```python
from build123d import *
from build123d.topology import SkipClean

# Parameters (mm, degrees)
SKETCH1_R           = 40
BOSS_EXTRUDE1_DEPTH = 4
BOSS_EXTRUDE2_DEPTH = 3
CUT_EXTRUDE1_DEPTH  = 3


with BuildPart() as part:
    # Sketch1 → Boss-Extrude1 (new body)
    with BuildSketch(Plane(origin=(0, 0, 0), x_dir=(1, 0, 0), z_dir=(0, 1, 0))):
        with Locations(Location((0, 0, 0), (0, 0, 270))):
            Circle(SKETCH1_R)
    extrude(amount=BOSS_EXTRUDE1_DEPTH)

    # Sketch2 → Boss-Extrude2 (add)
    with SkipClean():  # the faces are left unmerged after this step: merging them gives an invalid solid
        with BuildSketch(Plane(origin=(0, 4, 0), x_dir=(1, 0, 0), z_dir=(0, 1, 0))):
            with BuildLine():
                Line((70.838532525, 75.016207091), (33.556064162, 21.771324213))
                ThreePointArc((33.556064162, 21.771324213), (40, 0), (33.556064162, -21.771324213))
                Line((33.556064162, -21.771324213), (70.838532525, -75.016207091))
                ThreePointArc((70.838532525, -75.016207091), (67.154898406, -95.907134301), (46.263971196, -92.223500182))
                Line((46.263971196, -92.223500182), (8.981502833, -38.978617303))
                ThreePointArc((8.981502833, -38.978617303), (0, -40), (-8.981502833, -38.978617303))
                Line((-8.981502833, -38.978617303), (-46.263971196, -92.223500182))
                ThreePointArc((-46.263971196, -92.223500182), (-67.154898406, -95.907134301), (-70.838532525, -75.016207091))
                Line((-70.838532525, -75.016207091), (-33.556064162, -21.771324213))
                ThreePointArc((-33.556064162, -21.771324213), (-40, 0), (-33.556064162, 21.771324213))
                Line((-33.556064162, 21.771324213), (-70.838532525, 75.016207091))
                ThreePointArc((-70.838532525, 75.016207091), (-67.154898406, 95.907134301), (-46.263971196, 92.223500182))
                Line((-46.263971196, 92.223500182), (-8.981502833, 38.978617303))
                ThreePointArc((-8.981502833, 38.978617303), (0, 40), (8.981502833, 38.978617303))
                Line((8.981502833, 38.978617303), (46.263971196, 92.223500182))
                ThreePointArc((46.263971196, 92.223500182), (67.154898406, 95.907134301), (70.838532525, 75.016207091))
            make_face()
        extrude(amount=BOSS_EXTRUDE2_DEPTH)

    # Sketch3 → Cut-Extrude1 (cut)
    with SkipClean():  # the faces are left unmerged after this step: merging them gives an invalid solid
        with BuildSketch(Plane.XZ.offset(-4)):
            with BuildLine():
                Line((33.593734083, -37.516143596), (59.404673719, -74.377985589))
                ThreePointArc((59.404673719, -74.377985589), (57.931220071, -82.734356473), (49.574849188, -81.260902826))
                Line((49.574849188, -81.260902826), (23.763909552, -44.399060833))
                ThreePointArc((23.763909552, -44.399060833), (25.237363199, -36.042689949), (33.593734083, -37.516143596))
            make_face()
            with BuildLine():
                Line((-33.593734083, -37.516143596), (-59.404673719, -74.377985589))
                ThreePointArc((-59.404673719, -74.377985589), (-57.931220071, -82.734356473), (-49.574849188, -81.260902826))
                Line((-49.574849188, -81.260902826), (-23.763909552, -44.399060833))
                ThreePointArc((-23.763909552, -44.399060833), (-25.237363199, -36.042689949), (-33.593734083, -37.516143596))
            make_face()
            with BuildLine():
                Line((23.763909552, 44.399060833), (49.574849188, 81.260902826))
                ThreePointArc((49.574849188, 81.260902826), (57.931220071, 82.734356473), (59.404673719, 74.377985589))
                Line((59.404673719, 74.377985589), (33.593734083, 37.516143596))
                ThreePointArc((33.593734083, 37.516143596), (25.237363199, 36.042689949), (23.763909552, 44.399060833))
            make_face()
            with BuildLine():
                Line((-23.763909552, 44.399060833), (-49.574849188, 81.260902826))
                ThreePointArc((-49.574849188, 81.260902826), (-57.931220071, 82.734356473), (-59.404673719, 74.377985589))
                Line((-59.404673719, 74.377985589), (-33.593734083, 37.516143596))
                ThreePointArc((-33.593734083, 37.516143596), (-25.237363199, 36.042689949), (-23.763909552, 44.399060833))
            make_face()
        extrude(amount=-CUT_EXTRUDE1_DEPTH, mode=Mode.SUBTRACT)


solid = part.part
```
Design review of the part built by this model. Coordinates are the model's own, in mm. A direction names the side the tool comes from. Give positions to 0.01 mm unless a question says otherwise; leave off trailing zeros. Write each loop counter-clockwise with the first axis right and the second up, starting at its lowest first coordinate (ties: lowest second). Pieces come first, ordered by that corner, then holes.
(1) Add section D-D (z = 27). Give the boundary of the cut face in (x, y).
Checked values:
outline: (-37.22, 4) - (-29.51, 4) - (-29.51, 0) - (29.51, 0) - (29.51, 4) - (37.22, 4) - (37.22, 7) - (-37.22, 7) - close
(2) Add section A-A (x = 55.5). Give the boundary of the cut face in (y, z), and give its area (3 significant figures).
Checked values:
outline: (4, -98.31) - (7, -98.31) - (7, -83.73) - (4, -83.73) - close; (4, -68.8) - (7, -68.8) - (7, -53.11) - (4, -53.11) - close; (4, 53.11) - (7, 53.11) - (7, 68.8) - (4, 68.8) - close; (4, 83.73) - (7, 83.73) - (7, 98.31) - (4, 98.31) - close
area: 182 mm2
(3) Add section B-B (z = -48). Give the boundary of the cut face in (x, y).
Checked values:
outline: (-51.92, 4) - (-40.93, 4) - (-40.93, 7) - (-51.92, 7) - close; (-26.29, 4) - (-15.3, 4) - (-15.3, 7) - (-26.29, 7) - close; (15.3, 4) - (26.29, 4) - (26.29, 7) - (15.3, 7) - close; (40.93, 4) - (51.92, 4) - (51.92, 7) - (40.93, 7) - close
(4) Mouldability with a two-part tool opening along Z and no side actions: class faces 4 (the face through (-36.489, 5.479, 62.572)), 5 (the face through (27.9, 5.5, 66)), 6 (the face through (-36.85, 5.48, -63.09)), 7 (the face through (-27.9, 5.5, -66)) as +Z half, -Z half, draft (parallel to the pull), parting line (faces both ways), or undercut.
Checked values:
face 4: undercut
face 5: +Z half
face 6: undercut
face 7: -Z half
(5) Wall thickness on line 1 along X through (y, z) = (5.25, -78.5); line 2 along X through (y, z) = (4.25, 51); line 3 along Y through (x, z) = (42.5, 40): over which ranges is each line inside the solid? List them lowest first.
Checked values:
line 1: x = -72.65 to -60.45, -47.64 to -36.65, 36.65 to 47.64, 60.45 to 72.65
line 2: x = -54.02 to -43.04, -28.39 to -17.4, 17.4 to 28.39, 43.04 to 54.02
line 3: y = 4 to 7
(6) Clearance check with flat-ended pins moving along their axes: pin 1 Ø19.5 at (x, z) = (36.5, -67.5) entering from -Y; pin 2 Ø1 at (x, y) = (-0.5, 3) entering from -Z; pin 3 Ø3 at (x, y) = (-5, 4) entering from +Z. State where each tip first meets the part, or that it passes through.
Checked values:
pin 1: stops at y = 4
pin 2: stops at z = -40
pin 3: stops at z = 39.85
(7) Add section C-C (x = 36.5). Give the boundary of the cut face in (y, z).
Checked values:
outline: (0, -16.36) - (7, -16.36) - (7, 16.36) - (0, 16.36) - close; (4, -78.28) - (7, -78.28) - (7, -62.59) - (4, -62.59) - close; (4, -41.67) - (7, -41.67) - (7, -25.98) - (4, -25.98) - close; (4, 25.98) - (7, 25.98) - (7, 41.67) - (4, 41.67) - close; (4, 62.59) - (7, 62.59) - (7, 78.28) - (4, 78.28) - close
(8) Tool access review of faces 1 (the face through (27.362, 5.479, -65.228)), 2 (the face through (-27.362, 5.479, 65.228)), 3 (the face through (-51.936, 5.479, -48.021)): name each direction out of +Z, -Z, +X, -X, +Y, -Y from which nothing blocks a thin tool from reaching the whole face with its end or side.
Checked values:
face 1: -Z, +Y, -Y
face 2: +Z, +Y, -Y
face 3: -X, +Y, -Y
